```python
from build123d import *

# Parameters (mm, degrees)
SKETCH004_W      = 8.5
SKETCH004_H      = 2
SKETCH004_W_2    = 8
SKETCH004_W_3    = 2
SKETCH004_H_2    = 5.5
SKETCH004_H_3    = 6
SKETCH004_W_4    = 6.4
EXTRUDE001_DEPTH = 5
SKETCH002_R      = 1.5
PAD001_DEPTH     = 1.5
SKETCH003_R      = 3.5
SKETCH003_R_2    = 1.5
EXTRUDE_DEPTH    = 7.6


with BuildPart() as extrude001:
    # Sketch004 → Extrude001 (new body)
    with BuildSketch(Plane.XY):
        with Locations((-99.25, 46.7)):
            Rectangle(SKETCH004_W, SKETCH004_H)
        with Locations((99.25, 46.7)):
            Rectangle(SKETCH004_W, SKETCH004_H)
        with Locations((-99.5, -9.4)):
            Rectangle(SKETCH004_W_2, SKETCH004_H)
        with Locations((-83.5, -5.65)):
            Rectangle(SKETCH004_W_3, SKETCH004_H_2)
        with Locations((99.5, -9.4)):
            Rectangle(SKETCH004_W_2, SKETCH004_H)
        with Locations((83.5, -5.65)):
            Rectangle(SKETCH004_W_3, SKETCH004_H_2)
        with Locations((-75, 55)):
            Rectangle(SKETCH004_W_3, SKETCH004_H_3)
        with Locations((75, 55)):
            Rectangle(SKETCH004_W_3, SKETCH004_H_3)
        with Locations((-100.4, 21)):
            Rectangle(SKETCH004_W_4, SKETCH004_H)
        with Locations((100.4, 21)):
            Rectangle(SKETCH004_W_4, SKETCH004_H)
        with Locations((0, 68)):
            Rectangle(SKETCH004_W_3, SKETCH004_H_3)
    extrude(amount=EXTRUDE001_DEPTH)


with BuildPart() as body:
    # Sketch002 → Pad001 (new body)
    with BuildSketch(Plane.XY):
        with BuildLine():
            Line((-105.5, -52), (105.5, -52))
            Line((105.5, -52), (105.5, 50))
            ThreePointArc((105.5, 50), (98.763456, 66.263456), (82.5, 73))
            Line((-82.5, 73), (82.5, 73))
            ThreePointArc((-82.5, 73), (-98.763456, 66.263456), (-105.5, 50))
            Line((-105.5, -52), (-105.5, 50))
        make_face()
        with Locations((-95, -45)):
            Circle(SKETCH002_R, mode=Mode.SUBTRACT)
        with Locations((95, -45)):
            Circle(SKETCH002_R, mode=Mode.SUBTRACT)
        with BuildLine():
            Line((-14, -19.000009), (6, -19.000009))
            ThreePointArc((8, -21.000009), (7.414214, -19.585795), (6, -19.000009))
            Line((8, -21.000009), (8, -27.000009))
            Line((40, -27.000009), (8, -27.000009))
            ThreePointArc((42, -29.000009), (41.414214, -27.585795), (40, -27.000009))
            Line((42, -29.000009), (42, -50.000009))
            Line((24, -50.000009), (42, -50.000009))
            Line((24, -44.000009), (24, -50.000009))
            ThreePointArc((24, -44.000009), (23.414217, -42.58579), (22, -42))
            Line((22, -42), (9, -42))
            ThreePointArc((9, -42), (7.585783, -42.58579), (7, -44.000009))
            Line((7, -44.000009), (7, -50.000009))
            Line((-16, -50.000009), (7, -50.000009))
            Line((-16, -50.000009), (-16, -21.000009))
            ThreePointArc((-14, -19.000009), (-15.414214, -19.585795), (-16, -21.000009))
        make_face(mode=Mode.SUBTRACT)
        with BuildLine():
            ThreePointArc((-90, -37), (-90.707107, -37.292893), (-91, -38))
            Line((-91, -49), (-91, -38))
            ThreePointArc((-91, -49), (-90.707107, -49.707107), (-90, -50))
            Line((-79, -50), (-90, -50))
            ThreePointArc((-79, -50), (-78.292893, -49.707107), (-78, -49))
            Line((-78, -38), (-78, -49))
            ThreePointArc((-78, -38), (-78.292893, -37.292893), (-79, -37))
            Line((-90, -37), (-79, -37))
        make_face(mode=Mode.SUBTRACT)
        with BuildLine():
            ThreePointArc((91, -38), (90.707107, -37.292893), (90, -37))
            Line((90, -37), (79, -37))
            ThreePointArc((79, -37), (78.292893, -37.292893), (78, -38))
            Line((78, -38), (78, -49))
            ThreePointArc((78, -49), (78.292893, -49.707107), (79, -50))
            Line((79, -50), (90, -50))
            ThreePointArc((90, -50), (90.707107, -49.707107), (91, -49))
            Line((91, -49), (91, -38))
        make_face(mode=Mode.SUBTRACT)
    extrude(amount=-PAD001_DEPTH)


with BuildPart() as main:
    # Sketch003 → Extrude (new body)
    with BuildSketch(Plane.XY):
        with BuildLine():
            Line((-105.5, -52), (105.5, -52))
            Line((105.5, -52), (105.5, 50))
            ThreePointArc((105.5, 50), (98.763456, 66.263456), (82.5, 73))
            Line((-82.5, 73), (82.5, 73))
            ThreePointArc((-82.5, 73), (-98.763456, 66.263456), (-105.5, 50))
            Line((-105.5, -52), (-105.5, 50))
        make_face()
        with BuildLine():
            Line((-103.5, -50), (103.5, -50))
            Line((103.5, -50), (103.5, 50))
            ThreePointArc((103.5, 50), (97.349242, 64.849242), (82.5, 71))
            Line((-82.5, 71), (82.5, 71))
            ThreePointArc((-82.5, 71), (-97.349242, 64.849242), (-103.5, 50))
            Line((-103.5, -50), (-103.5, 50))
        make_face(mode=Mode.SUBTRACT)
        with Locations((-95, -45)):
            Circle(SKETCH003_R)
        with Locations((-95, -45)):
            Circle(SKETCH003_R_2, mode=Mode.SUBTRACT)
        with Locations((95, -45)):
            Circle(SKETCH003_R)
        with Locations((95, -45)):
            Circle(SKETCH003_R_2, mode=Mode.SUBTRACT)
        with Locations((-95, 55)):
            Circle(SKETCH003_R)
        with Locations((-95, 55)):
            Circle(SKETCH003_R_2, mode=Mode.SUBTRACT)
        with Locations((95, 55)):
            Circle(SKETCH003_R)
        with Locations((95, 55)):
            Circle(SKETCH003_R_2, mode=Mode.SUBTRACT)
        Polygon((-84.6, 44.1), (-82.6, 44.1), (-82.6, 50.1), (-69.6, 50.1), (-69.6, 52.1), (-84.6, 52.1), align=None)
        Polygon((84.6, 44.1), (82.6, 44.1), (82.6, 50.1), (69.6, 50.1), (69.6, 52.1), (84.6, 52.1), align=None)
    extrude(amount=EXTRUDE_DEPTH)

    # Fusion: union Body
    add(body.part)

    # Fusion001: union Extrude001
    add(extrude001.part)


solid = main.part
```
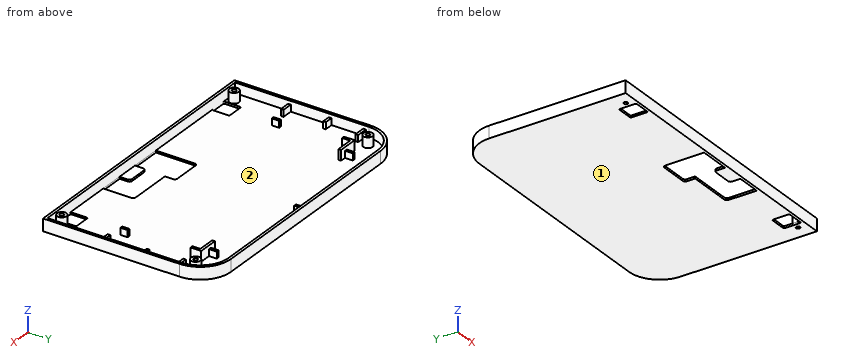
Verification items for the finished model (mm, model axes). Face numbers are marked on the shaded views. Coordinates: 2 decimals unless noted, no trailing zeros. Loops run counter-clockwise (first coordinate to the right, second up) from the corner with the lowest first, then second, coordinate; pieces in that order, holes last. Notation, with made-up numbers: (49.5, 47.25) -> (103.5, 47.25) arc R24 cw to (103.5, 65.25) -> close; hole circle Ø2 at (-26.75, 19). An arc over 180 degrees is marked (long way). Put each result on its own line as item: value.
1. Section check B-B, the plane y = 36. Record the boundary of the cut face in (x, z).
Result set:
outline: (-105.5, -1.5) -> (105.5, -1.5) -> (105.5, 7.6) -> (103.5, 7.6) -> (103.5, 0) -> (-103.5, 0) -> (-103.5, 7.6) -> (-105.5, 7.6) -> close
2. Section check C-C, the plane z = 2. Give the number of separate pieces and of enclosed holes in the cut face, then the cut area to 3 significant figures.
Result set:
separate pieces: 9
enclosed holes: 5
area: 1,650 mm^2
3. Mould release check, pull along X, two halves, no side actions. Record for the marked faces 1 and 2: pulls with the +X half, pulls with the -X half, needs draft (parallel to the pull), parting line crosses it, or undercut.
Result set:
face 1: needs draft
face 2: undercut
4. Thickness scan on line 1 (Y direction, x = -70.5, z = 3.5); line 2 (X direction, y = 43, z = 5); line 3 (X direction, y = 52, z = 3). Record the ranges inside material, lowest first.
Result set:
line 1: y = -52 to -50, 50.1 to 52.1, 71 to 73
line 2: x = -105.5 to -103.5, 103.5 to 105.5
line 3: x = -105.41 to -103.4, -96.8 to -93.2, -84.6 to -69.6, 69.6 to 84.6, 93.2 to 96.8, 103.4 to 105.41
5. Gauge pin test, flat ends, axial feed: P1, Ø1.6, axis at x = -83.5, z = 3.5, coming from the +Y side; P2, Ø1, axis at x = 83.5, y = -7, coming from the +Z side; P3, Ø6.5, axis at x = 18, y = -47.5, coming from the +Z side; P4, Ø12, axis at x = 40.5, y = 2.5, coming from the +Z side. Record the tip position at first contact, or that the pin passes through.
Result set:
P1: stops at y = 73
P2: stops at z = 5
P3: stops at z = 7.6
P4: stops at z = 0
